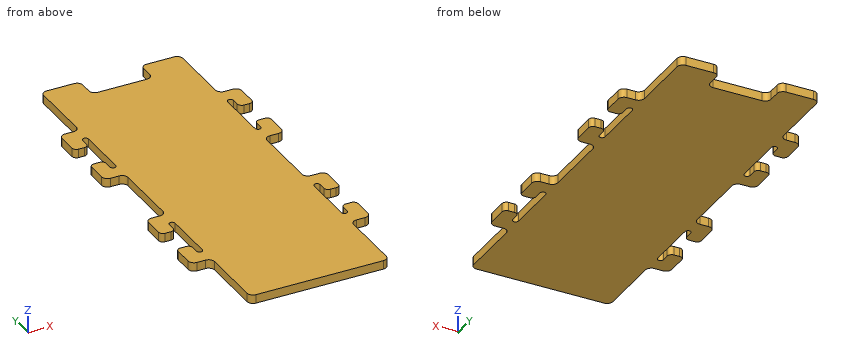
from build123d import *

# Parameters (mm, degrees)
F1_DEPTH = 3


with BuildPart() as f1:
    # F0 (on Top) → F1 (new body)
    with BuildSketch(Plane.XY):
        with BuildLine():
            ThreePointArc((0, 2), (0.585786, 0.585786), (2, 0))
            Line((2, 0), (24, 0))
            Line((24, 0), (46, 0))
            ThreePointArc((46, 0), (47.414214, 0.585786), (48, 2))
            Line((48, 2), (48, 23.5))
            ThreePointArc((48, 23.5), (48.585786, 24.914214), (50, 25.5))
            Line((50, 25.5), (53, 25.5))
            ThreePointArc((53, 25.5), (54.414214, 26.085786), (55, 27.5))
            Line((55, 27.5), (55, 34))
            ThreePointArc((55, 34), (54.56066, 35.06066), (53.5, 35.5))
            Line((53.5, 35.5), (51.5, 35.5))
            ThreePointArc((51.5, 35.5), (50.43934, 35.06066), (50, 34))
            Line((50, 34), (50, 31.5))
            ThreePointArc((50, 31.5), (49, 30.5), (48, 31.5))
            Line((48, 31.5), (48, 49.5))
            ThreePointArc((48, 49.5), (49, 50.5), (50, 49.5))
            Line((50, 49.5), (50, 47))
            ThreePointArc((50, 47), (50.43934, 45.93934), (51.5, 45.5))
            Line((51.5, 45.5), (53.5, 45.5))
            ThreePointArc((53.5, 45.5), (54.56066, 45.93934), (55, 47))
            Line((55, 47), (55, 53.5))
            ThreePointArc((55, 53.5), (54.414214, 54.914214), (53, 55.5))
            Line((53, 55.5), (50, 55.5))
            ThreePointArc((50, 55.5), (48.585786, 56.085786), (48, 57.5))
            Line((48, 57.5), (48, 80.5))
            ThreePointArc((48, 80.5), (48.585786, 81.914214), (50, 82.5))
            Line((50, 82.5), (53, 82.5))
            ThreePointArc((53, 82.5), (54.414214, 83.085786), (55, 84.5))
            Line((55, 84.5), (55, 91))
            ThreePointArc((55, 91), (54.56066, 92.06066), (53.5, 92.5))
            Line((53.5, 92.5), (51.5, 92.5))
            ThreePointArc((51.5, 92.5), (50.43934, 92.06066), (50, 91))
            Line((50, 91), (50, 88.5))
            ThreePointArc((50, 88.5), (49, 87.5), (48, 88.5))
            Line((48, 88.5), (48, 106.5))
            ThreePointArc((48, 106.5), (49, 107.5), (50, 106.5))
            Line((50, 106.5), (50, 104))
            ThreePointArc((50, 104), (50.43934, 102.93934), (51.5, 102.5))
            Line((51.5, 102.5), (53.5, 102.5))
            ThreePointArc((53.5, 102.5), (54.56066, 102.93934), (55, 104))
            Line((55, 104), (55, 110.5))
            ThreePointArc((55, 110.5), (54.414214, 111.914214), (53, 112.5))
            Line((53, 112.5), (50, 112.5))
            ThreePointArc((50, 112.5), (48.585786, 113.085786), (48, 114.5))
            Line((48, 114.5), (48, 136))
            ThreePointArc((48, 136), (47.414214, 137.414214), (46, 138))
            Line((46, 138), (36.5, 138))
            ThreePointArc((36.5, 138), (35.085786, 137.414214), (34.5, 136))
            Line((34.5, 136), (34.5, 132))
            ThreePointArc((34.5, 132), (33.914214, 130.585786), (32.5, 130))
            Line((32.5, 130), (24, 130))
            Line((24, 130), (15.5, 130))
            ThreePointArc((15.5, 130), (14.085786, 130.585786), (13.5, 132))
            Line((13.5, 132), (13.5, 136))
            ThreePointArc((13.5, 136), (12.914214, 137.414214), (11.5, 138))
            Line((11.5, 138), (2, 138))
            ThreePointArc((2, 138), (0.585786, 137.414214), (0, 136))
            Line((0, 136), (0, 114.5))
            ThreePointArc((0, 114.5), (-0.585786, 113.085786), (-2, 112.5))
            Line((-2, 112.5), (-5, 112.5))
            ThreePointArc((-5, 112.5), (-6.414214, 111.914214), (-7, 110.5))
            Line((-7, 110.5), (-7, 104))
            ThreePointArc((-7, 104), (-6.56066, 102.93934), (-5.5, 102.5))
            Line((-5.5, 102.5), (-3.5, 102.5))
            ThreePointArc((-3.5, 102.5), (-2.43934, 102.93934), (-2, 104))
            Line((-2, 104), (-2, 106.5))
            ThreePointArc((-2, 106.5), (-1, 107.5), (0, 106.5))
            Line((0, 106.5), (0, 88.5))
            ThreePointArc((0, 88.5), (-1, 87.5), (-2, 88.5))
            Line((-2, 88.5), (-2, 91))
            ThreePointArc((-2, 91), (-2.43934, 92.06066), (-3.5, 92.5))
            Line((-3.5, 92.5), (-5.5, 92.5))
            ThreePointArc((-5.5, 92.5), (-6.56066, 92.06066), (-7, 91))
            Line((-7, 91), (-7, 84.5))
            ThreePointArc((-7, 84.5), (-6.414214, 83.085786), (-5, 82.5))
            Line((-5, 82.5), (-2, 82.5))
            ThreePointArc((-2, 82.5), (-0.585786, 81.914214), (0, 80.5))
            Line((0, 80.5), (0, 57.5))
            ThreePointArc((0, 57.5), (-0.585786, 56.085786), (-2, 55.5))
            Line((-2, 55.5), (-5, 55.5))
            ThreePointArc((-5, 55.5), (-6.414214, 54.914214), (-7, 53.5))
            Line((-7, 53.5), (-7, 47))
            ThreePointArc((-7, 47), (-6.56066, 45.93934), (-5.5, 45.5))
            Line((-5.5, 45.5), (-3.5, 45.5))
            ThreePointArc((-3.5, 45.5), (-2.43934, 45.93934), (-2, 47))
            Line((-2, 47), (-2, 49.5))
            ThreePointArc((-2, 49.5), (-1, 50.5), (0, 49.5))
            Line((0, 49.5), (0, 31.5))
            ThreePointArc((0, 31.5), (-1, 30.5), (-2, 31.5))
            Line((-2, 31.5), (-2, 34))
            ThreePointArc((-2, 34), (-2.43934, 35.06066), (-3.5, 35.5))
            Line((-3.5, 35.5), (-5.5, 35.5))
            ThreePointArc((-5.5, 35.5), (-6.56066, 35.06066), (-7, 34))
            Line((-7, 34), (-7, 27.5))
            ThreePointArc((-7, 27.5), (-6.414214, 26.085786), (-5, 25.5))
            Line((-5, 25.5), (-2, 25.5))
            ThreePointArc((-2, 25.5), (-0.585786, 24.914214), (0, 23.5))
            Line((0, 23.5), (0, 2))
        make_face()
    extrude(amount=F1_DEPTH)


solid = f1.part
Check sheet for the modelled part. Datum: model origin and axes. Units: mm. Give positions to 0.01 mm unless a question says otherwise; leave off trailing zeros. Write each loop counter-clockwise with the first axis right and the second up, starting at its lowest first coordinate (ties: lowest second). Pieces come first, ordered by that corner, then holes. Notation, with made-up numbers: (3.25, -0.75) -> (49.25, -0.75) arc R24 ccw to (49.25, 20.25) -> close; hole circle Ø9 at (17.25, 85.5). An arc over 180 degrees is marked (long way). One line per item, written item: value. Start each with the question number.
Item 1: Gauge pin test, flat ends, axial feed: pin 1 (0.9 mm diameter, centred on x = 51.5, z = 1.5, fed in from +Y); pin 2 (0.9 mm diameter, centred on x = 26.5, z = 1, fed in from +Y); pin 3 (3 mm diameter, centred on x = 34, y = 23, fed in from -Z); pin 4 (0.6 mm diameter, centred on x = 52.5, z = 2, fed in from -Y). Record the tip position at first contact, or that the pin passes through.
Item 2: Section check A-A on y = 122.5. Record the cut outline in (x, z).
Item 3: Material ranges on probe 1 along Y at (x, z) = (-3.5, 1.4); probe 2 along X at (y, z) = (64.5, 0.75); probe 3 along Y at (x, z) = (-3, 0.2), recorded low to high. Write a range as from..to.
Results list:
1. pin 1: y = 112.5
1. pin 2: y = 130
1. pin 3: z = 0
1. pin 4: y = 25.5
2. outline: (0, 0) -> (48, 0) -> (48, 3) -> (0, 3) -> close
3. probe 1: 25.5..35.5, 45.5..55.5, 82.5..92.5, 102.5..112.5
3. probe 2: 0..48
3. probe 3: 25.5..35.41, 45.59..55.5, 82.5..92.41, 102.59..112.5
